Verification items for the finished model (mm, model axes). Give positions to 0.01 mm unless a question says otherwise; leave off trailing zeros. Order: outer loops, then holes, each group sorted by start corner. A loop starts at its lowest first (then second) coordinate and runs counter-clockwise, first axis right, second up.
from build123d import *

# Parameters (mm, degrees)
SKETCH1_W           = 87.63
SKETCH1_H           = 80
BOSS_EXTRUDE1_DEPTH = 5
SKETCH2_R           = 2.075
SKETCH2_R_2         = 1.85
CUT_EXTRUDE1_DEPTH  = 6
CUT_EXTRUDE2_REACH  = 7
SKETCH3_R           = 2.2
CUT_EXTRUDE3_REACH  = 7


with BuildPart() as part:
    # Sketch1 → Boss-Extrude1 (new body)
    with BuildSketch(Plane(origin=(0, 0, 0), x_dir=(1, 0, 0), z_dir=(0, 1, 0))):
        with Locations((43.815, 40)):
            Rectangle(SKETCH1_W, SKETCH1_H)
    extrude(amount=BOSS_EXTRUDE1_DEPTH)

    # Sketch2 → Cut-Extrude1 (cut, through all)
    with BuildSketch(Plane(origin=(0, 5, 0), x_dir=(1, 0, 0), z_dir=(0, 1, 0))):
        with Locations(Location((12.465, 70.4, 0), (0, 0, 270))):  # turned: the seam where the file's is
            Circle(SKETCH2_R)
        with Locations(Location((12.465, 20.4, 0), (0, 0, 270))):  # turned: the seam where the file's is
            Circle(SKETCH2_R)
        with Locations(Location((14.465, 40, 0), (0, 0, 270))):  # turned: the seam where the file's is
            Circle(SKETCH2_R_2)
        with Locations(Location((73.165, 40, 0), (0, 0, 270))):  # turned: the seam where the file's is
            Circle(SKETCH2_R_2)
        with Locations(Location((75.165, 9.6, 0), (0, 0, 270))):  # turned: the seam where the file's is
            Circle(SKETCH2_R)
        with Locations(Location((75.165, 59.6, 0), (0, 0, 270))):  # turned: the seam where the file's is
            Circle(SKETCH2_R)
    extrude(amount=-CUT_EXTRUDE1_DEPTH, mode=Mode.SUBTRACT)

    # Sketch3 → Cut-Extrude2 (cut, up to next)
    with BuildSketch(Plane(origin=(0, 5, 0), x_dir=(1, 0, 0), z_dir=(0, 1, 0)), mode=Mode.PRIVATE) as cut_extrude2_sk1:
        with Locations(Location((43.81, 55.25, 0), (0, 0, 270))):  # turned: the seam where the file's is
            Circle(SKETCH3_R)
    cut_extrude2_tool1 = extrude(cut_extrude2_sk1.sketch, amount=-CUT_EXTRUDE2_REACH, mode=Mode.PRIVATE) & part.part
    add(cut_extrude2_tool1.solids().sort_by_distance((43.81, 5, -55.25))[0], mode=Mode.SUBTRACT)
    # Sketch3 → Cut-Extrude2 (cut, up to next)
    with BuildSketch(Plane(origin=(0, 5, 0), x_dir=(1, 0, 0), z_dir=(0, 1, 0)), mode=Mode.PRIVATE) as cut_extrude2_sk2:
        with Locations(Location((43.82, 24.75, 0), (0, 0, 270))):  # turned: the seam where the file's is
            Circle(SKETCH3_R)
    cut_extrude2_tool2 = extrude(cut_extrude2_sk2.sketch, amount=-CUT_EXTRUDE2_REACH, mode=Mode.PRIVATE) & part.part
    add(cut_extrude2_tool2.solids().sort_by_distance((43.82, 5, -24.75))[0], mode=Mode.SUBTRACT)

    # Sketch4 → Cut-Extrude3 (cut, up to next)
    with BuildSketch(Plane(origin=(0, 5, 0), x_dir=(1, 0, 0), z_dir=(0, 1, 0)), mode=Mode.PRIVATE) as cut_extrude3_sk1:
        with BuildLine():
            Line((38.21, 60), (38.21, 20))
            ThreePointArc((38.21, 20), (33.81, 15.6), (29.41, 20))
            Line((29.41, 20), (29.41, 60))
            ThreePointArc((29.41, 60), (33.81, 64.4), (38.21, 60))
        make_face()
    cut_extrude3_tool1 = extrude(cut_extrude3_sk1.sketch, amount=-CUT_EXTRUDE3_REACH, mode=Mode.PRIVATE) & part.part
    add(cut_extrude3_tool1.solids().sort_by_distance((33.81, 5, -40))[0], mode=Mode.SUBTRACT)
    # Sketch4 → Cut-Extrude3 (cut, up to next)
    with BuildSketch(Plane(origin=(0, 5, 0), x_dir=(1, 0, 0), z_dir=(0, 1, 0)), mode=Mode.PRIVATE) as cut_extrude3_sk2:
        with BuildLine():
            Line((58.21, 60), (58.21, 20))
            ThreePointArc((58.21, 20), (53.81, 15.6), (49.41, 20))
            Line((49.41, 20), (49.41, 60))
            ThreePointArc((49.41, 60), (53.81, 64.4), (58.21, 60))
        make_face()
    cut_extrude3_tool2 = extrude(cut_extrude3_sk2.sketch, amount=-CUT_EXTRUDE3_REACH, mode=Mode.PRIVATE) & part.part
    add(cut_extrude3_tool2.solids().sort_by_distance((53.81, 5, -40))[0], mode=Mode.SUBTRACT)


solid = part.part
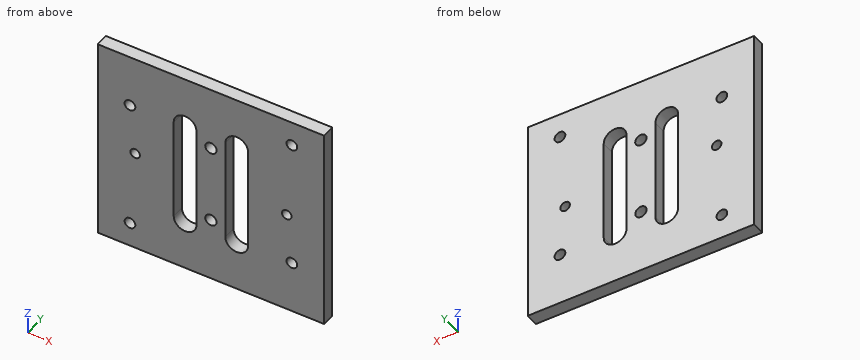
(1) Section check C-C, the plane z = -55.25. Enter the section's corners in (x, y).
Solved:
outline: (0, 0) - (29.41, 0) - (29.41, 5) - (0, 5) - close; (38.21, 0) - (41.61, 0) - (41.61, 5) - (38.21, 5) - close; (46.01, 0) - (49.41, 0) - (49.41, 5) - (46.01, 5) - close; (58.21, 0) - (87.63, 0) - (87.63, 5) - (58.21, 5) - close
(2) Scan lines: line 1 (X direction, y = 0.7, z = -20.5); line 2 (X direction, y = 2.85, z = -44); line 3 (X direction, y = 3.15, z = -55.25). Record each from-to range of solid material in increasing order.
Solved:
line 1: x = 0 to 10.39, 14.54 to 29.41, 38.21 to 49.41, 58.21 to 87.63
line 2: x = 0 to 29.41, 38.21 to 49.41, 58.21 to 87.63
line 3: x = 0 to 29.41, 38.21 to 41.61, 46.01 to 49.41, 58.21 to 87.63
(3) Section check B-B, the plane x = 53.81. Enter the section's corners in (y, z), then the cut area to 3 significant figures.
Solved:
outline: (0, -80) - (5, -80) - (5, -64.4) - (0, -64.4) - close; (0, -15.6) - (5, -15.6) - (5, 0) - (0, 0) - close
area: 156 mm2
(4) Section check D-D, the plane y = 1.3. Give the number of separate pieces and of enclosed holes in the cut face, then the cut area to 3 significant figures.
Solved:
separate pieces: 1
enclosed holes: 10
area: 6,080 mm2
(5) Go/stop test with a flat-tipped pin: pin 1 (2.5 mm diameter, centred on x = 75.165, z = -9.6, fed in from -Y). Record where the tip stops, or that it passes through.
Solved:
pin 1: passes through
(6) Section check A-A, the plane z = -9.6. Enter the section's corners in (x, y), then the cut area to 3 significant figures.
Solved:
outline: (0, 0) - (73.09, 0) - (73.09, 5) - (0, 5) - close; (77.24, 0) - (87.63, 0) - (87.63, 5) - (77.24, 5) - close
area: 417 mm2
